Source: CAD feature listing. Evaluate the final solid. Frame: model axes, mm. Round coordinates to 2 decimals unless told otherwise and drop trailing zeros. Loops run counter-clockwise (first coordinate to the right, second up) from the corner with the lowest first, then second, coordinate; pieces in that order, holes last. Notation, with made-up numbers: (-15.75, 29) -> (39.25, 29) arc R23 cw to (39.25, 63) -> close; hole circle Ø2 at (-33.5, 86). An arc over 180 degrees is marked (long way). Write item = value, one per line.
from build123d import *

# Parameters (mm, degrees)
F0_W        = 38.1
F0_H        = 3.0734
F1_DEPTH    = 10.16
F3_T1_DEPTH = 61.4345004446
F4_DEPTH    = 25.4


# Not quite as in the source:
# - a fillet or chamfer that OpenCascade refuses, or shapes differently, is made with other operations: its cross-section is extruded or revolved along the edge and cut away or added


with BuildPart() as f1:
    # F0 (on Top) → F1 (new body)
    with BuildSketch(Plane.XY):
        with Locations((0, 1.5367)):
            Rectangle(F0_W, F0_H)
    extrude(amount=F1_DEPTH)

    # F3: fillet of radius 5.08 on 1 edges, made by hand

    # F3_s2 → F3_t1 (cut)
    with BuildSketch(Plane.YZ.offset(-30.7172502223)):
        with BuildLine():
            ThreePointArc((3.0734, 5.4930999111), (2.2360364445, 8.2870999111), (0, 10.16))
            Line((0, 10.16), (3.0734, 10.16))
            Line((3.0734, 10.16), (3.0734, 5.4930999111))
        make_face()
    extrude(amount=F3_T1_DEPTH, mode=Mode.SUBTRACT)

    # F2 (on face) → F4 (cut)
    with BuildSketch(Plane.XZ):
        Polygon((-15.875, 8.7222954744), (-15.0449409051, 10.16), (-16.7050590949, 10.16), align=None)
        Polygon((-4.7382939367, 10.16), (-6.6917060633, 10.16), (-5.715, 8.4682954744), align=None)
        Polygon((6.5450590949, 10.16), (4.8849409051, 10.16), (5.715, 8.7222954744), align=None)
        Polygon((16.7050590949, 10.16), (15.0449409051, 10.16), (15.875, 8.7222954744), align=None)
    extrude(amount=-F4_DEPTH, mode=Mode.SUBTRACT)


solid = f1.part
1. Section query D-D (y = 2.7). Return the cut outline in (x, z), then the cut area to 3 significant figures.
Evaluation:
outline = (-19.05, 0) -> (19.05, 0) -> (19.05, 7.4) -> (-19.05, 7.4) -> close
area = 282 mm²
2. Contact query for a flat-ended pin moving along its axis: pin 1 Ø4 at (x, z) = (-4, 4.5) entering from -Y. Output: stop coordinate, or through.
Evaluation:
pin_1 = 0
3. Mould query, pull axis X, two halves, no side actions, for faces 1 (the face through (-19.05, 2, 5)), 2 (the face through (0, 2, 0)), 3 (the face through (-6.102, 0.806, 9.138)). Classes: released by +X, released by -X, zero draft, split by the parting line, or undercut.
Evaluation:
face_1 = released by -X
face_2 = zero draft
face_3 = undercut
4. Section query B-B (x = 10). Return the cut outline in (y, z).
Evaluation:
outline = (0, 0) -> (3.07, 0) -> (3.07, 5.49) arc R5.08 ccw to (0, 10.16) -> close
5. Line query: probe 1 along Y at (x, z) = (1, 5.75); probe 2 along Z at (x, y) = (8, 0.35); probe 3 along Z at (x, y) = (-15.5, 1.05). Output: solid intervals per line, ascending. Write a range as from..to.
Evaluation:
probe_1 = 0..3.07
probe_2 = 0..9.99
probe_3 = 0..9.37
6. Section query A-A (y = 0.95). Return the cut outline in (x, z) (3 decimals).
Evaluation:
outline = (-19.05, 0) -> (19.05, 0) -> (19.05, 9.624) -> (16.396, 9.624) -> (15.875, 8.722) -> (15.354, 9.624) -> (6.236, 9.624) -> (5.715, 8.722) -> (5.194, 9.624) -> (-5.048, 9.624) -> (-5.715, 8.468) -> (-6.382, 9.624) -> (-15.354, 9.624) -> (-15.875, 8.722) -> (-16.396, 9.624) -> (-19.05, 9.624) -> close
7. Section query C-C (x = -15.5). Return the cut outline in (y, z), then the cut area to 3 significant figures.
Evaluation:
outline = (0, 0) -> (3.07, 0) -> (3.07, 5.49) arc R5.08 ccw to (1.27, 9.37) -> (0, 9.37) -> close
area = 26.7 mm²
